from build123d import *

# Parameters (mm, degrees)
SKETCH1_R           = 6.731
BOSS_EXTRUDE1_DEPTH = 17.4752
SKETCH2_W           = 2.1971
SKETCH2_H           = 10.16
SKETCH3_R           = 1.5875
CUT_EXTRUDE1_DEPTH  = 17.4752


with BuildPart() as part:
    # Sketch1 → Boss-Extrude1 (new body)
    with BuildSketch(Plane(origin=(0, 0, 0), x_dir=(1, 0, 0), z_dir=(0, 1, 0))):
        with Locations(Location((0, 0, 0), (0, 0, 270))):
            Circle(SKETCH1_R)
    extrude(amount=BOSS_EXTRUDE1_DEPTH)

    # Sketch2 → Cut-Revolve1 (revolve, cut)
    with BuildSketch(Plane(origin=(0, 0, 0), x_dir=(0, 0, -1), z_dir=(1, 0, 0)), mode=Mode.PRIVATE) as cut_revolve1_sk:
        with Locations((5.63245, 11.43)):
            Rectangle(SKETCH2_W, SKETCH2_H)
    revolve(cut_revolve1_sk.sketch.rotate(Axis((0, 18.309331677, 0), (0, -1, 0)), 180), axis=Axis((0, 18.309331677, 0), (0, -1, 0)), mode=Mode.SUBTRACT)

    # Sketch3 → Cut-Extrude1 (cut)
    with BuildSketch(Plane(origin=(0, 17.4752, 0), x_dir=(1, 0, 0), z_dir=(0, 1, 0))):
        with Locations(Location((0, 0, 0), (0, 0, 270))):
            Circle(SKETCH3_R)
    extrude(amount=-CUT_EXTRUDE1_DEPTH, mode=Mode.SUBTRACT)


solid = part.part
Input: part model. Units: mm. Frame: model coordinates. A direction names the side the tool comes from. Round coordinates to 2 decimals unless told otherwise and drop trailing zeros. Loops run counter-clockwise (first coordinate to the right, second up) from the corner with the lowest first, then second, coordinate; pieces in that order, holes last. Notation, with made-up numbers: (67.25, 47.25) -> (113.25, 47.25) arc R22 cw to (113.25, 66.25) -> close; hole circle Ø7 at (36, 83.25). An arc over 180 degrees is marked (long way). Answer as a JSON object with one key per item and string values. Group by question number.
1) Draft query along Z for faces 1 (the flat face through (2, 17.475, 0)), 2 (the cylindrical face through (-0.966, 8.86, -1.26)), 3 (the cylindrical face through (5.676, 3.131, 3.619)). Return one class per face: +Z half, -Z half, draft (parallel to the pull), parting line (faces both ways), or undercut.
2) Section query D-D on x = 5.75. Output: boundary loops of the cut face in (y, z).
3) Reachability of faces 4 (the cylindrical face through (5.676, 16.986, 3.619)), 5 (the flat face through (-5, 6.35, 0)) from +Z, -Z, +X, -X, +Y, -Y: full face, straight path, thin tool, end or side. Return the list, or none.
4) Section query B-B on z = 0. Output: boundary loops of the cut face in (x, y).
5) Ray query, L1, parallel to Y at x = -3.25, z = 3.5; L2, parallel to X at y = 13.75, z = 0; L3, parallel to X at y = 5, z = 0. Return the intervals inside material, ascending.
6) Pin query (flat end, axial travel): pin 1 (6 mm diameter, centred on x = 4.5, y = 12.5, fed in from -Z); pin 2 (3 mm diameter, centred on x = 2.5, y = 13, fed in from +Z); pin 3 (2 mm diameter, centred on y = 12, z = -4.5, fed in from -X); pin 4 (2.5 mm diameter, centred on x = 0, z = 0, fed in from -Y). Return the tip coordinate at first contact, or that it passes through.
7) Section query C-C on y = 4. Output: boundary loops of the cut face in (x, z) (1 decimal).
8) Section query A-A on x = 0. Output: boundary loops of the cut face in (y, z).
Reply:
{
 "1": {"face 1": "draft", "face 2": "undercut", "face 3": "parting line"},
 "2": {"outline": "(0, -3.5) -> (6.35, -3.5) -> (6.35, 3.5) -> (0, 3.5) -> close; (16.51, -3.5) -> (17.48, -3.5) -> (17.48, 3.5) -> (16.51, 3.5) -> close"},
 "3": {"face 4": "+Y, -Y", "face 5": "none"},
 "4": {"outline": "(-6.73, 0) -> (-1.59, 0) -> (-1.59, 17.48) -> (-6.73, 17.48) -> (-6.73, 16.51) -> (-4.53, 16.51) -> (-4.53, 6.35) -> (-6.73, 6.35) -> close; (1.59, 0) -> (6.73, 0) -> (6.73, 6.35) -> (4.53, 6.35) -> (4.53, 16.51) -> (6.73, 16.51) -> (6.73, 17.48) -> (1.59, 17.48) -> close"},
 "5": {"L1": "y = 0 to 6.35, 16.51 to 17.48", "L2": "x = -4.53 to -1.59, 1.59 to 4.53", "L3": "x = -6.73 to -1.59, 1.59 to 6.73"},
 "6": {"pin 1": "stops at z = -4.28", "pin 2": "stops at z = 4.42", "pin 3": "stops at x = -2.88", "pin 4": "passes through"},
 "7": {"outline": "circle Ø13.5 at (0, 0); hole circle Ø3.2 at (0, 0)"},
 "8": {"outline": "(0, -6.73) -> (6.35, -6.73) -> (6.35, -4.53) -> (16.51, -4.53) -> (16.51, -6.73) -> (17.48, -6.73) -> (17.48, -1.59) -> (0, -1.59) -> close; (0, 1.59) -> (17.48, 1.59) -> (17.48, 6.73) -> (16.51, 6.73) -> (16.51, 4.53) -> (6.35, 4.53) -> (6.35, 6.73) -> (0, 6.73) -> close"}
}
